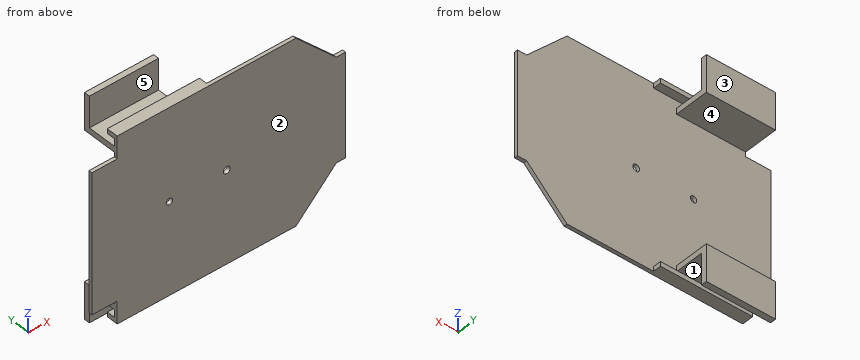
Autodesk Inventor part; units mm, degrees
ref_plane "YZ Plane" through (0, 0, 0) normal (1, 0, 0) x (0, 1, 0)
ref_plane "XZ Plane" through (0, 0, 0) normal (0, 1, 0) x (-1, 0, 0)
ref_plane "XY Plane" through (0, 0, 0) normal (0, 0, 1) x (1, 0, 0)
sketch "Skizze1" plane through (0, 0, 0) normal (0, 1, 0) x (-1, 0, 0)
  circle A0 centre (-117, -80) radius 3
  circle A1 centre (-67.25, -80) radius 2.75
  line L0 (-170, -160) -> (-22, -160)
  line L1 (-220, -125) -> (-212, -125)
  line L2 (-212, -35) -> (-220, -35)
  line L3 (-220, -35) -> (-220, -125)
  line L4 (0, -19.5) -> (-22, -19.5)
  line L5 (-212, -35) -> (-177, 0)
  line L6 (-212, -125) -> (-177, -160)
  line L7 (-22, -140.5) -> (0, -140.5)
  line L8 (-22, 0) -> (-22, -15.5)
  line L9 (-22, -19.5) -> (0, -19.5)
  line L10 (-22, -160) -> (-22, -144.5)
  line L11 (-22, -140.5) -> (0, -140.5)
  line L12 (-22, 0) -> (-102, 0)
  line L13 (-102, 0) -> (-102, -4)
  line L14 (-22, -15.5) -> (-22, 0)
  line L15 (-22, -160) -> (-102, -160)
  line L16 (-102, -160) -> (-102, -156)
  line L17 (-22, -144.5) -> (-22, -160)
  line L18 (-22, -160) -> (-102, -160)
  line L19 (-102, -160) -> (-102, -156)
  line L20 (-102, -156) -> (-22, -156)
  line L21 (-22, -156) -> (-22, -160)
  line L22 (-22, -156) -> (-102, -156)
  line L23 (-22, -149.5) -> (-22, -156)
  line L24 (-22, 0) -> (-102, 0)
  line L25 (-102, 0) -> (-102, -4)
  line L26 (-102, -4) -> (-22, -4)
  line L27 (-22, -4) -> (-22, 0)
  line L28 (-22, -4) -> (-102, -4)
  line L29 (-22, -10.5) -> (-22, -4)
  line L30 (-22, -15.5) -> (-22, -10.5)
  line L31 (-22, -149.5) -> (-82, -149.5)
  line L32 (-22, -144.5) -> (-22, -149.5)
  line L33 (-22, -144.5) -> (-22, -140.5)
  line L34 (-22, 0) -> (-177, 0)
  line L35 (-22, 0) -> (-170, 0)
  line L36 (-22, -15.5) -> (-22, -19.5)
  line L37 (0, -19.5) -> (0, -140.5)
  line L38 (-22, -144.5) -> (-82, -144.5)
  line L39 (-82, -144.5) -> (-82, -149.5)
  line L40 (-82, -149.5) -> (-22, -149.5)
  line L41 (-22, -149.5) -> (-22, -144.5)
  line L42 (-22, -15.5) -> (-82, -15.5)
  line L43 (-82, -15.5) -> (-82, -10.5)
  line L44 (-82, -10.5) -> (-22, -10.5)
  line L45 (-22, -10.5) -> (-22, -15.5)
  line L46 (-82, -15.5) -> (-22, -15.5)
  line L47 (-82, -144.5) -> (-22, -144.5)
  line L48 (-82, -10.5) -> (-22, -10.5)
  line L49 (-220, -35) -> (-220, -125)
  line L50 (-177, -160) -> (-22, -160)
  point P0 (0, 0)
  point P1 (-216, -125)
  point P2 (-216, -35)
  point P3 (-22, -4)
  dimension "d4" = 6
  dimension "d5" = 49.75
  dimension "d7" = 5.5
  dimension "d9" = 8
  dimension "d10" = 90
  dimension "d14" = 60.5
  dimension "d15" = 60.5
  dimension "d17" = 35
  dimension "d25" = 4
  dimension "d27" = 4
  dimension "d31" = 60
  dimension "d32" = 60
extrude "Extrusion1" add sketch "Skizze1" along normal blind 3 contours L50 L6 L1 L3 L2 L5 L34 L13 L26 L8 L44 L43 L42 L36 L4 L37 L7 L33 L38 L39 L31 L10 L20 L16 L0
sketch "Skizze2" plane through (0, 0, 0) normal (0, -1, 0) x (1, 0, 0)
  line L0 (22, -15.5) -> (82, -15.5)
  line L1 (82, -15.5) -> (82, -10.5)
  line L2 (22, -15.5) -> (82, -15.5)
  line L3 (82, -15.5) -> (82, -10.5)
  line L4 (82, -10.5) -> (22, -10.5)
  line L5 (22, -10.5) -> (22, -15.5)
  line L6 (22, -149.5) -> (82, -149.5)
  line L7 (82, -144.5) -> (22, -144.5)
  line L8 (22, -149.5) -> (82, -149.5)
  line L9 (82, -149.5) -> (82, -144.5)
  line L10 (82, -144.5) -> (22, -144.5)
  line L11 (22, -144.5) -> (22, -149.5)
  line L12 (102, -156) -> (22, -156)
  line L13 (177, -160) -> (102, -160)
  line L14 (22, -156) -> (102, -156)
  line L15 (102, -156) -> (102, -160)
  line L16 (102, -160) -> (22, -160)
  line L17 (22, -160) -> (22, -156)
  line L18 (22, -4) -> (102, -4)
  line L19 (102, 0) -> (177, 0)
  line L20 (22, -4) -> (102, -4)
  line L21 (102, -4) -> (102, 0)
  line L22 (102, 0) -> (22, 0)
  line L23 (22, 0) -> (22, -4)
  point P0 (0, 0)
extrude "Extrusion2" add sketch "Skizze2" against normal blind 10 contours L15 L16 L17 L12 | L23 L22 L21 L18
sketch "Skizze3" plane through (0, 0, 0) normal (0, -1, 0) x (1, 0, 0)
  line L0 (82, -15.5) -> (82, -10.5)
  line L1 (22, -15.5) -> (82, -15.5)
  line L2 (82, -15.5) -> (82, -10.5)
  line L3 (82, -10.5) -> (22, -10.5)
  line L4 (22, -10.5) -> (22, -15.5)
  line L5 (82, -144.5) -> (22, -144.5)
  line L6 (82, -149.5) -> (82, -144.5)
  line L7 (22, -144.5) -> (82, -144.5)
  line L8 (82, -144.5) -> (82, -149.5)
  line L9 (82, -149.5) -> (22, -149.5)
  line L10 (22, -149.5) -> (22, -144.5)
  point P0 (0, 0)
extrude "Extrusion3" add sketch "Skizze3" against normal blind 33
sketch "Skizze4" plane through (22, 3, -10.5) normal (0, 0, 1) x (1, 0, 0)
  line L0 (0, 0) -> (0, 30)
  line L1 (60, 0) -> (60, 30)
  line L2 (0, 30) -> (60, 30)
  line L3 (60, 30) -> (60, 25)
  line L4 (60, 25) -> (0, 25)
  line L5 (0, 25) -> (0, 30)
  point P0 (-22, -3)
  dimension "d39" = 5
extrude "Extrusion4" add sketch "Skizze4" along normal blind 27
sketch "Skizze5" plane through (82, 3, -149.5) normal (0, 0, -1) x (-1, 0, 0)
  line L0 (0, 0) -> (0, 30)
  line L1 (60, 0) -> (60, 30)
  line L2 (0, 30) -> (60, 30)
  line L3 (60, 30) -> (60, 25)
  line L4 (60, 25) -> (0, 25)
  line L5 (0, 25) -> (0, 30)
  point P0 (82, -3)
  dimension "d42" = 5
extrude "Extrusion5" add sketch "Skizze5" along normal blind 27
properties part number "boschprofil-platform"
Input: part model. Units: mm. Frame: model coordinates. Face numbers are marked on the shaded views. A direction names the side the tool comes from. Give positions to 0.01 mm unless a question says otherwise; leave off trailing zeros. Write each loop counter-clockwise with the first axis right and the second up, starting at its lowest first coordinate (ties: lowest second). Pieces come first, ordered by that corner, then holes. Notation, with made-up numbers: M 79.25,74 L 136.25,74 A17 ccw 136.25,86 Z; hole C -17.5,-15 d4. An arc over 180 degrees is marked long. Write item = value, one per line. Start each with the question number.
1) Draft query along Y for the marked faces 3, 4 and 5. Return one class per face: +Y half, -Y half, draft (parallel to the pull), parting line (faces both ways), or undercut.
2) First-contact query: pin 1 Ø2 at (x, y) = (74, 5) entering from +Z; pin 2 Ø1 at (x, z) = (144, -36) entering from +Y; pin 3 Ø3 at (y, z) = (5.5, -1) entering from +X. Flat tips, straight axial feed; report the tip coordinate or a pass-through.
3) Cut plane D-D on y = 20. Return the cut outline in (x, z), then the cut area to 3 significant figures.
4) Cut plane C-C on y = 7. Return the cut outline in (x, z).
5) Cut plane A-A on x = 117. Return the cut outline in (y, z).
6) Cut plane B-B on z = -80. Return the cut outline in (x, y), then the cut area to 4 significant figures.
7) Material intervals for line 1 along Z through (x, y) = (67.25, 1.8); line 2 along Z through (x, y) = (46.5, 31); line 3 along Y through (x, z) = (91.5, -120), sorted ascending. Write a range as [from, to].
8) Reachability of the marked faces 1 and 2 from +Z, -Z, +X, -X, +Y, -Y: full face, straight path, thin tool, end or side. Return the list, or none.
Solved:
q1.face_3 = +Y half
q1.face_4 = draft
q1.face_5 = undercut
q2.pin_1 = 0
q2.pin_2 = 3
q2.pin_3 = 102
q3.outline = M 22,-149.5 L 82,-149.5 L 82,-144.5 L 22,-144.5 Z; M 22,-15.5 L 82,-15.5 L 82,-10.5 L 22,-10.5 Z
q3.area = 600 mm2
q4.outline = M 22,-160 L 102,-160 L 102,-156 L 22,-156 Z; M 22,-149.5 L 82,-149.5 L 82,-144.5 L 22,-144.5 Z; M 22,-15.5 L 82,-15.5 L 82,-10.5 L 22,-10.5 Z; M 22,-4 L 102,-4 L 102,0 L 22,0 Z
q5.outline = M 0,-160 L 3,-160 L 3,-83 L 0,-83 Z; M 0,-77 L 3,-77 L 3,0 L 0,0 Z
q6.outline = M 0,0 L 64.5,0 L 64.5,3 L 0,3 Z; M 70,0 L 114,0 L 114,3 L 70,3 Z; M 120,0 L 220,0 L 220,3 L 120,3 Z
q6.area = 625.5 mm2
q7.line_1 = [-160, -82.75], [-77.25, 0]
q7.line_2 = [-176.5, -144.5], [-15.5, 16.5]
q7.line_3 = [0, 3]
q8.face_1 = +X, -X
q8.face_2 = +Z, -Z, +X, -X, -Y
